Work out the finished part from the listing and answer in its coordinate system (mm). A direction names the side the tool comes from. Give positions to 0.01 mm unless a question says otherwise; leave off trailing zeros. Loops run counter-clockwise (first coordinate to the right, second up) from the corner with the lowest first, then second, coordinate; pieces in that order, holes last. Notation, with made-up numbers: (-21.5, -18.5) - (18.5, -18.5) arc R12 ccw to (18.5, -7.5) - close; hole circle Ø4 at (56.25, -22.75). An arc over 180 degrees is marked (long way). One line per question, with ' | ' between items. Start each with the question number.
1. Section B-B (y = 3.64) is taken. Determine the outline of the cut face in (x, z).
2. For a pull along Z with two mould halves and no side action, classify faces 3 (the face through (5, 3, -13.7)), 4 (the face through (5, 3, 0)), 5 (the face through (6, 3, -4.3)) as released by +Z, released by -Z, zero draft, split by the parting line, or undercut.
3. Section A-A (x = 4.5) is taken. Determine the outline of the cut face in (y, z).
4. Which of the six approach directions +Z, -Z, +X, -X, +Y, -Y give full straight-line access (tool end or side, diameter ignored) to faces 1 (the face through (2.5, 3, -7)), 2 (the face through (10, 3, -12))?
5. Find the intervals of material crossed by line 1 (Z direction, x = 3, y = 2.45); line 2 (X direction, y = 3.05, z = -9); line 3 (X direction, y = 1.5, z = -4), in increasing order.
6. Section C-C (z = -12) is taken. Determine the outline of the cut face in (x, y), plus the area to 3 significant figures.
7. Section D-D (y = 0.3) is taken. Determine the outline of the cut face in (x, z).
8. This flat-tipped pin is pushed along its axis until it touches: pin 1 (1.5 mm diameter, centred on y = 3, z = -6.5, fed in from -X). Where does it stop, or does it pass through?
from build123d import *

# Parameters (mm, degrees)
BOSS_EXTRUDE1_DEPTH = 5.2
SKETCH2_R           = 0.3
BOSS_EXTRUDE2_DEPTH = 5.2


with BuildPart() as part:
    # Sketch1 → Boss-Extrude1 (new body)
    with BuildSketch(Plane(origin=(0, 0, 0), x_dir=(1, 0, 0), z_dir=(0, 1, 0))):
        Polygon((0, 0), (0, 13.7), (10, 13.7), (10, 9.4), (2.5, 9.4), (2.5, 4.3), (10, 4.3), (10, 0), align=None)
    extrude(amount=BOSS_EXTRUDE1_DEPTH)

    # Sketch2 → Boss-Extrude2 (add)
    with BuildSketch(Plane.ZY):
        with Locations(Location((-12, 3.64, 0), (0, 0, 180))):
            Circle(SKETCH2_R)
        with Locations(Location((-1.7, 3.64, 0), (0, 0, 180))):
            Circle(SKETCH2_R)
        with Locations(Location((-1.7, 1.56, 0), (0, 0, 180))):
            Circle(SKETCH2_R)
        with Locations(Location((-12, 1.56, 0), (0, 0, 180))):
            Circle(SKETCH2_R)
    extrude(amount=BOSS_EXTRUDE2_DEPTH)


solid = part.part
Conclusion:
1) outline: (-5.2, -12.3) - (0, -12.3) - (0, -13.7) - (10, -13.7) - (10, -9.4) - (2.5, -9.4) - (2.5, -4.3) - (10, -4.3) - (10, 0) - (0, 0) - (0, -1.4) - (-5.2, -1.4) - (-5.2, -2) - (0, -2) - (0, -11.7) - (-5.2, -11.7) - close
2) face 3: released by -Z | face 4: released by +Z | face 5: undercut
3) outline: (0, -13.7) - (5.2, -13.7) - (5.2, -9.4) - (0, -9.4) - close; (0, -4.3) - (5.2, -4.3) - (5.2, 0) - (0, 0) - close
4) face 1: +X, +Y, -Y | face 2: +Z, -Z, +X, +Y, -Y
5) line 1: -13.7 to -9.4, -4.3 to 0 | line 2: 0 to 2.5 | line 3: 0 to 10
6) outline: (-5.2, 1.26) - (0, 1.26) - (0, 0) - (10, 0) - (10, 5.2) - (0, 5.2) - (0, 3.94) - (-5.2, 3.94) - (-5.2, 3.34) - (0, 3.34) - (0, 1.86) - (-5.2, 1.86) - close | area: 58.2 mm²
7) outline: (0, -13.7) - (10, -13.7) - (10, -9.4) - (2.5, -9.4) - (2.5, -4.3) - (10, -4.3) - (10, 0) - (0, 0) - close
8) pin 1: x = 0
